Geometry: see drawing. Coordinates: mm, zero at the bounding-box minimum. Give positions to 0.01 mm unless a question says otherwise; leave off trailing zeros. Write each loop counter-clockwise with the first axis right and the second up, starting at its lowest first coordinate (ties: lowest second). Pieces come first, ordered by that corner, then holes. Notation, with made-up numbers: (19, -31) - (27, -31) arc R24 cw to (27, -4) - close; hole circle Ø5 at (19.5, 58.25). An arc over 180 degrees is marked (long way). Use a Markdown table: item, result. Add a question column.
1. Material intervals for probe 1 along Z at (x, y) = (11.5, 22.5); probe 2 along Y at (x, z) = (12, 10.5); probe 3 along X at (y, z) = (14.75, 32), sorted ascending.
2. Section query A-A, the plane x = 12. Return loops of the section in (y, z), plus the area to 3 significant figures.
3. Pin query (flat end, axial travel): pin 1 (8 mm diameter, centred on x = 11.5, z = 28, fed in from +Y); pin 2 (6 mm diameter, centred on x = 18, z = 21.5, fed in from -Y); pin 3 (6 mm diameter, centred on x = 6, z = 18.5, fed in from +Y). Return the tip coordinate at first contact, or that it passes through.
4. Section query C-C, the plane z = 20. Return loops of the section in (x, y).
5. Mould query, pull axis Z, two halves, no side actions, for the marked faces 1, 2 and 3. Classes: released by +Z, released by -Z, zero draft, split by the parting line, or undercut.
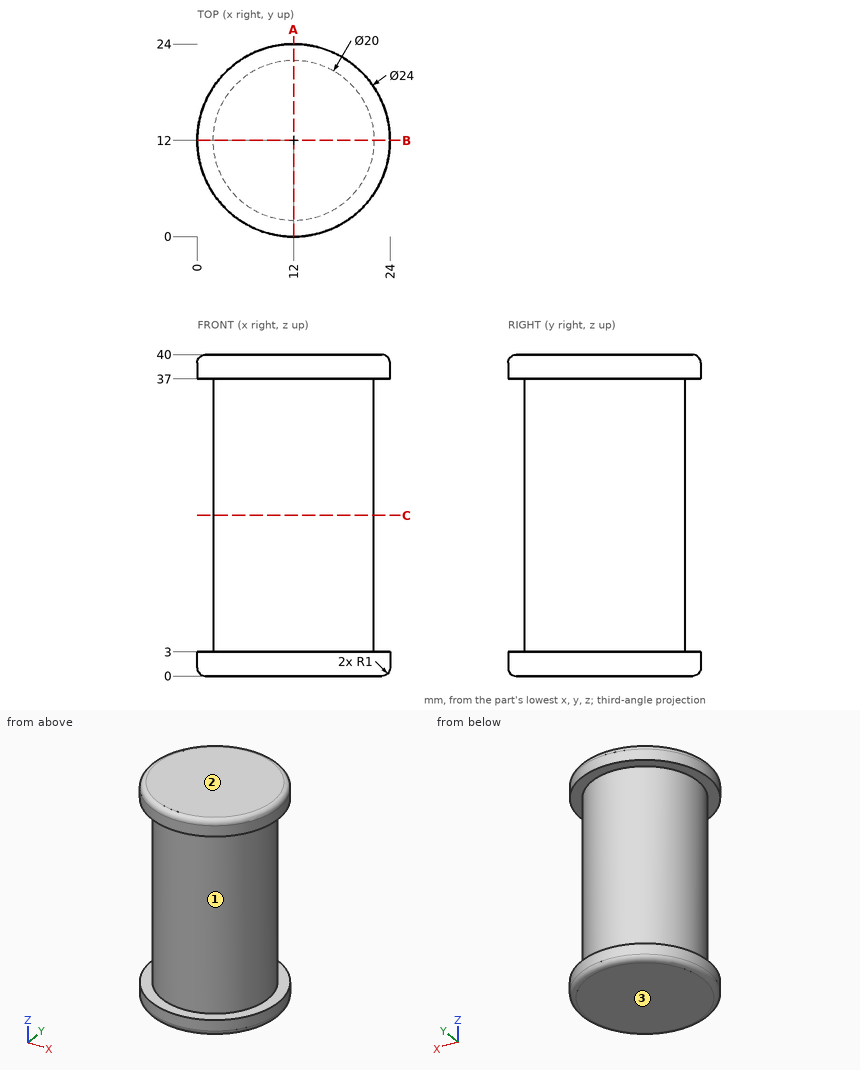
Result sheet:
| question | item | result |
|---|---|---|
| 1 | probe 1 | z = 0 to 3, 37 to 40 |
| 1 | probe 2 | y = 2 to 22 |
| 1 | probe 3 | x = 2.39 to 21.61 |
| 2 | outline | (0, 1) arc R1 ccw to (1, 0) - (23, 0) arc R1 ccw to (24, 1) - (24, 3) - (22, 3) - (22, 37) - (24, 37) - (24, 39) arc R1 ccw to (23, 40) - (1, 40) arc R1 ccw to (0, 39) - (0, 37) - (2, 37) - (2, 3) - (0, 3) - close |
| 2 | area | 823 mm² |
| 3 | pin 1 | stops at y = 22 |
| 3 | pin 2 | stops at y = 2.46 |
| 3 | pin 3 | stops at y = 21.54 |
| 4 | outline | circle Ø20 at (12, 12) |
| 5 | face 1 | undercut |
| 5 | face 2 | released by +Z |
| 5 | face 3 | released by -Z |
